Build history of the part. All positions in model axes, mm. A direction names the side the tool comes from. Round coordinates to 2 decimals unless told otherwise and drop trailing zeros. Loops run counter-clockwise (first coordinate to the right, second up) from the corner with the lowest first, then second, coordinate; pieces in that order, holes last. Notation, with made-up numbers: (79, 33) - (122, 33) arc R34 cw to (122, 72) - close; hole circle Ø3 at (-31, 55.5). An arc over 180 degrees is marked (long way). One line per question, with ' | ' between items. Start each with the question number.
from build123d import *

# Parameters (mm, degrees)
CROQUIS1_W              = 50.8
CROQUIS1_H              = 6.31
SALIENTE_EXTRUIR1_DEPTH = 273.99
CROQUIS2_W              = 50.8
CROQUIS2_H              = 6.31
SALIENTE_EXTRUIR2_DEPTH = 772.95
CROQUIS3_W              = 50.8
CROQUIS3_H              = 6.31
SALIENTE_EXTRUIR3_DEPTH = 324.39
CROQUIS4_R              = 4.7625
CORTAR_EXTRUIR1_DEPTH   = 10
CROQUIS5_R              = 6.5
CORTAR_EXTRUIR2_DEPTH   = 10
CROQUIS6_R              = 5
CORTAR_EXTRUIR3_DEPTH   = 35


with BuildPart() as part:
    # Croquis1 → Saliente-Extruir1 (new body)
    with BuildSketch(Plane.XY):
        Rectangle(CROQUIS1_W, CROQUIS1_H)
    extrude(amount=SALIENTE_EXTRUIR1_DEPTH)

    # Croquis2 → Saliente-Extruir2 (add)
    with BuildSketch(Plane(origin=(0, 3.155, 0), x_dir=(1, 0, 0), z_dir=(0, 1, 0))):
        with Locations((0, -270.835)):
            Rectangle(CROQUIS2_W, CROQUIS2_H)
    extrude(amount=SALIENTE_EXTRUIR2_DEPTH)

    # Croquis3 → Saliente-Extruir3 (add)
    with BuildSketch(Plane(origin=(0, 0, 267.68), x_dir=(-1, 0, 0), z_dir=(0, 0, -1))):
        with Locations((0, 772.95)):
            Rectangle(CROQUIS3_W, CROQUIS3_H)
    extrude(amount=SALIENTE_EXTRUIR3_DEPTH)

    # Croquis4 → Cortar-Extruir1 (cut)
    with BuildSketch(Plane.XZ.offset(3.155)):
        with Locations((-12.7, 12.7)):
            Circle(CROQUIS4_R)
        with Locations((12.7, 38.1)):
            Circle(CROQUIS4_R)
    extrude(amount=-CORTAR_EXTRUIR1_DEPTH, mode=Mode.SUBTRACT)

    # Croquis5 → Cortar-Extruir2 (cut)
    with BuildSketch(Plane(origin=(0, 776.105, 0), x_dir=(1, 0, 0), z_dir=(0, 1, 0))):
        with Locations(Location((0, 40.21, 0), (0, 0, 180))):
            Circle(CROQUIS5_R)
        with Locations(Location((0, 9.21, 0), (0, 0, 180))):
            Circle(CROQUIS5_R)
    extrude(amount=-CORTAR_EXTRUIR2_DEPTH, mode=Mode.SUBTRACT)

    # Croquis6 → Cortar-Extruir3 (cut)
    with BuildSketch(Plane(origin=(0, 776.105, 0), x_dir=(1, 0, 0), z_dir=(0, 1, 0))):
        with Locations(Location((0, -187.48, 0), (0, 0, 180))):
            Circle(CROQUIS6_R)
    extrude(amount=-CORTAR_EXTRUIR3_DEPTH, mode=Mode.SUBTRACT)


solid = part.part
1) Saw through at A-A on y = 707. Write the cut outline in (x, z).
2) Tool access for faces 1 (the flat face through (0, 769.795, 108)), 2 (the flat face through (0, -3.155, 135)): list every direction of +Z, -Z, +X, -X, +Y, -Y with a clear straight run to the whole face (end or side of a thin tool).
3) Wall check: line 1 (Z direction, x = 0, y = 773.75); line 2 (Y direction, x = 22, z = 207) (3 decimals); line 3 (X direction, y = -1, z = 38). Give the ranges that are in metal, low to high. Write a range as [from, to].
4) Two-plate mould, pull along Y, no slides. Class faces 3 (the flat face through (0, 3.155, 132)), 4 (the flat face through (25.4, 385, 269)), 5 (the flat face through (0, 776.105, 111)), 6 (the flat face through (0, 381, 267.68)): +Y half, -Y half, draft (parallel to the pull), parting line (faces both ways), or undercut.
5) Drop flat-ended pins along their axis: pin 1 (5.5 mm diameter, centred on x = -12.7, z = 12.7, fed in from -Y) (3 decimals); pin 2 (7 mm diameter, centred on x = 4.5, y = -1, fed in from -Z); pin 3 (5 mm diameter, centred on x = 7.5, y = 491, fed in from -Z). Give the stop position or say it passes through.
Answer key:
1) outline: (-25.4, 267.68) - (25.4, 267.68) - (25.4, 273.99) - (-25.4, 273.99) - close
2) face 1: -Z, +X, -X | face 2: +Z, -Z, +X, -X, -Y
3) line 1: [-56.71, -46.71], [-33.71, -15.71], [-2.71, 182.48], [192.48, 273.99] | line 2: [-3.155, 3.155], [769.795, 776.105] | line 3: [-25.4, 7.94], [17.46, 25.4]
4) face 3: undercut | face 4: draft | face 5: +Y half | face 6: undercut
5) pin 1: y = 769.795 | pin 2: z = 0 | pin 3: z = 267.68
